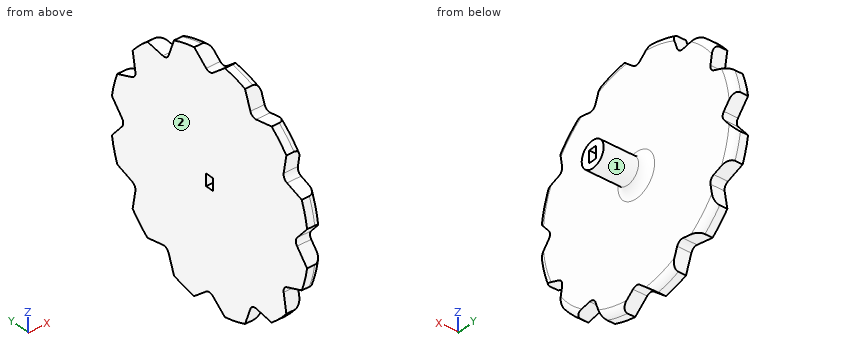
```python
from build123d import *

# Parameters (mm, degrees)
BOSS_EXTRUDE1_DEPTH = 6.5
SKETCH2_R           = 6
BOSS_EXTRUDE2_DEPTH = 20
FILLET1_R           = 3
SKETCH3_W           = 5.5
SKETCH3_H           = 3.81
CUT_EXTRUDE1_DEPTH  = 27.5000001
FILLET2_R           = 4


with BuildPart() as part:
    # Sketch1 → Boss-Extrude1 (new body)
    with BuildSketch(Plane(origin=(0, 0, 0), x_dir=(0, 0, -1), z_dir=(1, 0, 0))):
        with BuildLine():
            Line((1.815874997, 47.835924448), (8.381939498, 53.345506749))
            ThreePointArc((8.381939498, 53.345506749), (13.976228436, 52.15999462), (19.413780836, 50.389533771))
            Line((19.413780836, 50.389533771), (22.345368346, 42.335063284))
            ThreePointArc((22.345368346, 42.335063284), (23.5875, 40.854748424), (25.490556102, 40.519188287))
            Line((25.490556102, 40.519188287), (33.931725912, 42.007594273))
            ThreePointArc((33.931725912, 42.007594273), (38.183766184, 38.183766184), (42.007594273, 33.931725912))
            Line((42.007594273, 33.931725912), (40.519188287, 25.490556102))
            ThreePointArc((40.519188287, 25.490556102), (40.854748424, 23.5875), (42.335063284, 22.345368346))
            Line((42.335063284, 22.345368346), (50.389533771, 19.413780836))
            ThreePointArc((50.389533771, 19.413780836), (52.15999462, 13.976228436), (53.345506749, 8.381939498))
            Line((53.345506749, 8.381939498), (47.835924448, 1.815874997))
            ThreePointArc((47.835924448, 1.815874997), (47.175, 0), (47.835924448, -1.815874997))
            Line((47.835924448, -1.815874997), (53.345506749, -8.381939498))
            ThreePointArc((53.345506749, -8.381939498), (52.15999462, -13.976228436), (50.389533771, -19.413780836))
            Line((50.389533771, -19.413780836), (42.335063284, -22.345368346))
            ThreePointArc((42.335063284, -22.345368346), (40.854748424, -23.5875), (40.519188287, -25.490556102))
            Line((40.519188287, -25.490556102), (42.007594273, -33.931725912))
            ThreePointArc((42.007594273, -33.931725912), (38.183766184, -38.183766184), (33.931725912, -42.007594273))
            Line((33.931725912, -42.007594273), (25.490556102, -40.519188287))
            ThreePointArc((25.490556102, -40.519188287), (23.5875, -40.854748424), (22.345368346, -42.335063284))
            Line((22.345368346, -42.335063284), (19.413780836, -50.389533771))
            ThreePointArc((19.413780836, -50.389533771), (13.976228436, -52.15999462), (8.381939498, -53.345506749))
            Line((8.381939498, -53.345506749), (1.815874997, -47.835924448))
            ThreePointArc((1.815874997, -47.835924448), (0, -47.175), (-1.815874997, -47.835924448))
            Line((-1.815874997, -47.835924448), (-8.381939498, -53.345506749))
            ThreePointArc((-8.381939498, -53.345506749), (-13.976228436, -52.15999462), (-19.413780836, -50.389533771))
            Line((-19.413780836, -50.389533771), (-22.345368346, -42.335063284))
            ThreePointArc((-22.345368346, -42.335063284), (-23.5875, -40.854748424), (-25.490556102, -40.519188287))
            Line((-25.490556102, -40.519188287), (-33.931725912, -42.007594273))
            ThreePointArc((-33.931725912, -42.007594273), (-38.183766184, -38.183766184), (-42.007594273, -33.931725912))
            Line((-42.007594273, -33.931725912), (-40.519188287, -25.490556102))
            ThreePointArc((-40.519188287, -25.490556102), (-40.854748424, -23.5875), (-42.335063284, -22.345368346))
            Line((-42.335063284, -22.345368346), (-50.389533771, -19.413780836))
            ThreePointArc((-50.389533771, -19.413780836), (-52.15999462, -13.976228436), (-53.345506749, -8.381939498))
            Line((-53.345506749, -8.381939498), (-47.835924448, -1.815874997))
            ThreePointArc((-47.835924448, -1.815874997), (-47.175, 0), (-47.835924448, 1.815874997))
            Line((-47.835924448, 1.815874997), (-53.345506749, 8.381939498))
            ThreePointArc((-53.345506749, 8.381939498), (-52.15999462, 13.976228436), (-50.389533771, 19.413780836))
            Line((-50.389533771, 19.413780836), (-42.335063284, 22.345368346))
            ThreePointArc((-42.335063284, 22.345368346), (-40.854748424, 23.5875), (-40.519188287, 25.490556102))
            Line((-40.519188287, 25.490556102), (-42.007594273, 33.931725912))
            ThreePointArc((-42.007594273, 33.931725912), (-38.183766184, 38.183766184), (-33.931725912, 42.007594273))
            Line((-33.931725912, 42.007594273), (-25.490556102, 40.519188287))
            ThreePointArc((-25.490556102, 40.519188287), (-23.5875, 40.854748424), (-22.345368346, 42.335063284))
            Line((-22.345368346, 42.335063284), (-19.413780836, 50.389533771))
            ThreePointArc((-19.413780836, 50.389533771), (-13.976228436, 52.15999462), (-8.381939498, 53.345506749))
            Line((-8.381939498, 53.345506749), (-1.815874997, 47.835924448))
            ThreePointArc((-1.815874997, 47.835924448), (0, 47.175), (1.815874997, 47.835924448))
        make_face()
    extrude(amount=BOSS_EXTRUDE1_DEPTH)

    # Sketch2 → Boss-Extrude2 (add)
    with BuildSketch(Plane(origin=(6.5, 0, 0), x_dir=(0, 0, -1), z_dir=(1, 0, 0))):
        Circle(SKETCH2_R)
    extrude(amount=BOSS_EXTRUDE2_DEPTH)

    # Fillet1
    fillet1_edges = [part.edges().sort_by_distance(p)[0] for p in [
        (6.5, -52.15999462, 13.976228436),
        (6.5, -52.15999462, -13.976228436),
        (6.5, 52.15999462, -13.976228436),
        (6.5, -38.183766184, -38.183766184),
        (6.5, -13.976228436, -52.15999462),
        (6.5, 13.976228436, -52.15999462),
        (6.5, 38.183766184, -38.183766184),
        (6.5, 52.15999462, 13.976228436),
        (6.5, 38.183766184, 38.183766184),
        (6.5, 13.976228436, 52.15999462),
        (6.5, -13.976228436, 52.15999462),
        (6.5, -38.183766184, 38.183766184),
    ]]
    fillet(fillet1_edges, radius=FILLET1_R)

    # Sketch3 → Cut-Extrude1 (cut, through all)
    with BuildSketch(Plane(origin=(26.5, 0, 0), x_dir=(0, 0, -1), z_dir=(1, 0, 0))):
        Rectangle(SKETCH3_W, SKETCH3_H)
    extrude(amount=-CUT_EXTRUDE1_DEPTH, mode=Mode.SUBTRACT)

    # Fillet2
    fillet2_edges = [part.edges().sort_by_distance(p)[0] for p in [
        (6.5, 0, 6),
    ]]
    fillet(fillet2_edges, radius=FILLET2_R)


solid = part.part
```
Work out the finished part from the listing and answer in its coordinate system (mm). Face numbers are marked on the shaded views. A direction names the side the tool comes from. Give positions to 0.01 mm unless a question says otherwise; leave off trailing zeros. Loops run counter-clockwise (first coordinate to the right, second up) from the corner with the lowest first, then second, coordinate; pieces in that order, holes last. Notation, with made-up numbers: (65, 70.25) -> (72, 70.25) arc R5 cw to (72, 79.25) -> close; hole circle Ø2 at (42.25, 19.5). An arc over 180 degrees is marked (long way). Use CSV: the item, a comma, the result in double quotes.
1. The part is cut by section B-B (z = 0). Write down the section's boundary in (x, y) (3 decimals).
Found:
outline,"(0, -47.175) -> (6.5, -47.175) -> (6.5, -10) arc R4 cw to (10.5, -6) -> (26.5, -6) -> (26.5, -1.905) -> (0, -1.905) -> close; (0, 1.905) -> (26.5, 1.905) -> (26.5, 6) -> (10.5, 6) arc R4 cw to (6.5, 10) -> (6.5, 47.175) -> (0, 47.175) -> close"
2. Flat-ended cylindrical pins translate along their axes: pin 1 Ø8 at (x, z) = (6, 17) entering from +Y; pin 2 Ø3 at (x, z) = (18, 1) entering from -Y; pin 3 Ø5 at (y, z) = (1, -18.5) entering from +X. Find the tip coordinate at first contact, or state that the pin passes through.
Found:
pin 1,"y = 52.23"
pin 2,"y = -6"
pin 3,"x = 6.5"
3. The part is cut by section D-D (z = 44). Write down the section's boundary in (x, y).
Found:
outline,"(0, -21.74) -> (6.5, -21.74) -> (6.5, 21.74) -> (0, 21.74) -> close"
4. Straight lines are drawn through the part: line 1 (X direction, y = -45, z = -13); line 2 (Y direction, x = 12.75, z = -1) (3 decimals); line 3 (Y direction, x = 1.75, z = -14.5). For each, find the intervals that lie inside material, in ascending order.
Found:
line 1,"0 to 6.5"
line 2,"-5.916 to -1.905, 1.905 to 5.916"
line 3,"-52.02 to 52.02"
5. The part is cut by section A-A (y = 0). Write down the section's boundary in (x, z) (3 decimals).
Found:
outline,"(0, -47.175) -> (6.5, -47.175) -> (6.5, -10) arc R4 cw to (10.5, -6) -> (26.5, -6) -> (26.5, -2.75) -> (0, -2.75) -> close; (0, 2.75) -> (26.5, 2.75) -> (26.5, 6) -> (10.5, 6) arc R4 cw to (6.5, 10) -> (6.5, 47.175) -> (0, 47.175) -> close"
6. A tool of negligible diameter and unlimited length cuts with its end or side. For the marked faces 1 and 2, from which of +Z, -Z, +X, -X, +Y, -Y can it reach the whole face along a straight path? Write none if from no direction.
Found:
face 1,"+X"
face 2,"+Z, -Z, -X, +Y, -Y"
7. The part is cut by section C-C (x = 14.5). Write down the section's boundary in (y, z) (3 decimals).
Found:
outline,"circle Ø12 at (0, 0); hole (-1.905, -2.75) -> (1.905, -2.75) -> (1.905, 2.75) -> (-1.905, 2.75) -> close"
